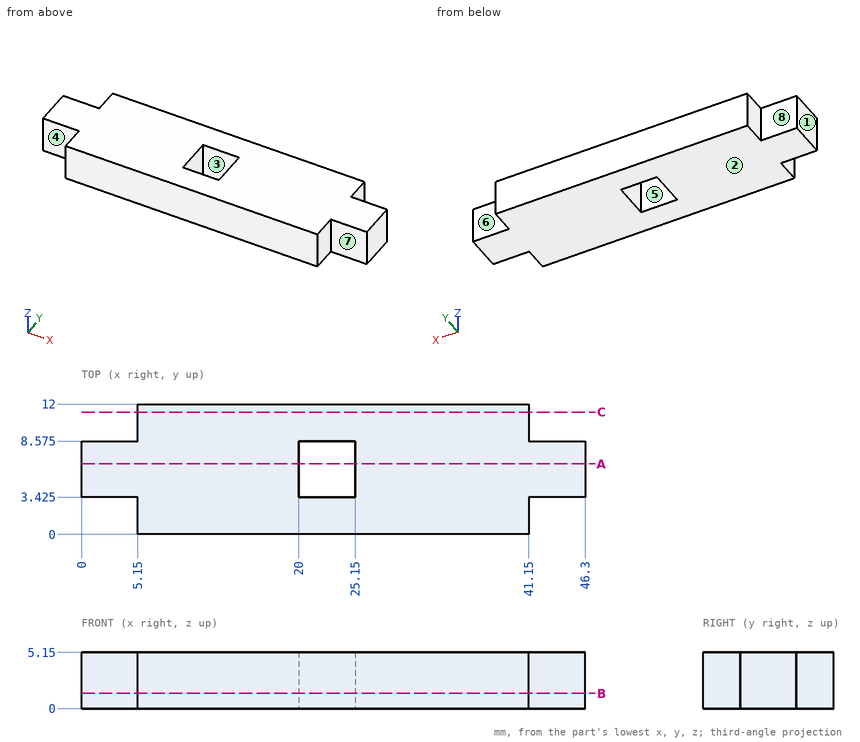
Check sheet for the drawn part. Datum: minimum x, y, z corner. Units: mm. A direction names the side the tool comes from. Give positions to 0.01 mm unless a question says otherwise; leave off trailing zeros. Loops run counter-clockwise (first coordinate to the right, second up) from the corner with the lowest first, then second, coordinate; pieces in that order, holes last.
1) Draft check along X on the marked faces 1, 2 and 3. Enter one of: pulls with the +X half, pulls with the -X half, needs draft (parallel to the pull), parting line crosses it, or undercut.
2) Sectioned sample at C-C, the plane y = 11.25. Enter the section's corners in (x, z), then the cut area to 3 significant figures.
3) Sectioned sample at A-A, the plane y = 6.5. Enter the section's corners in (x, z), then the cut area to 3 significant figures.
4) Set-up check for the marked faces 4, 5, 6, 7 and 8: record each of +Z, -Z, +X, -X, +Y, -Y from which the full face is reachable in a straight line by a thin tool's end or side.
5) Sectioned sample at B-B, the plane z = 1.4. Enter the section's corners in (x, y) (3 decimals), then the cut area to 3 significant figures.
6) Thickness scan on line 1 along X through (y, z) = (6, 4); line 2 along Y through (x, z) = (42, 3.6) (3 decimals); line 3 along X through (y, z) = (2.5, 4.5). Record the ranges inside material, lowest first.
7) Depth check by flat-ended pin: pin 1 Ø2.5 at (y, z) = (1, 3.5) entering from +X; pin 2 Ø1 at (y, z) = (10.5, 3) entering from -X; pin 3 Ø2.5 at (x, z) = (42.5, 3) entering from +Y (3 decimals). Enter the tip coordinate at first touch or a pass-through.
Answers:
1. face 1: pulls with the -X half
1. face 2: needs draft
1. face 3: undercut
2. outline: (5.15, 0) - (41.15, 0) - (41.15, 5.15) - (5.15, 5.15) - close
2. area: 185 mm2
3. outline: (0, 0) - (20, 0) - (20, 5.15) - (0, 5.15) - close; (25.15, 0) - (46.3, 0) - (46.3, 5.15) - (25.15, 5.15) - close
3. area: 212 mm2
4. face 4: +Z, -Z, -X, -Y
4. face 5: +Z, -Z
4. face 6: +Z, -Z, +X, +Y
4. face 7: +Z, -Z, +X, -Y
4. face 8: +Z, -Z, -X, +Y
5. outline: (0, 3.425) - (5.15, 3.425) - (5.15, 0) - (41.15, 0) - (41.15, 3.425) - (46.3, 3.425) - (46.3, 8.575) - (41.15, 8.575) - (41.15, 12) - (5.15, 12) - (5.15, 8.575) - (0, 8.575) - close; hole (20, 3.425) - (25.15, 3.425) - (25.15, 8.575) - (20, 8.575) - close
5. area: 459 mm2
6. line 1: x = 0 to 20, 25.15 to 46.3
6. line 2: y = 3.425 to 8.575
6. line 3: x = 5.15 to 41.15
7. pin 1: stops at x = 41.15
7. pin 2: stops at x = 5.15
7. pin 3: stops at y = 8.575
